Drawing for the job (mm, zero at the part's lowest x, y, z). Coordinates: 2 decimals unless noted, no trailing zeros. Write each loop counter-clockwise with the first axis right and the second up, starting at its lowest first coordinate (ties: lowest second). Pieces come first, ordered by that corner, then holes. Notation, with made-up numbers: M 31,42.25 L 81,42.25 A23 ccw 81,77.25 Z; hole C 67.25,24.5 d6. An arc over 180 degrees is marked long. Put each result on its own line as item: value. Start each with the question number.
Q1. Cut at B-B (x = 81). Write the cut outline in (y, z).
Q2. Cut at A-A (z = 70). Write the cut outline in (x, y).
Q3. Drill centre lines: line 1 along X through (y, z) = (5, 35); line 2 along Z through (x, y) = (208, 3.75); line 3 along Z through (x, y) = (134.57, 4). Where is each one in solid material? Low to high.
Q4. Drop a flat-ended pin along its axis: pin 1 (4 mm diameter, centred on x = 208, z = 35, fed in from +Y). Give the stop position or say it passes through.
Q5. Cut at C-C (x = 134.57). Write the cut outline in (y, z).
Q6. Cut at D-D (z = 35). Write the cut outline in (x, y).
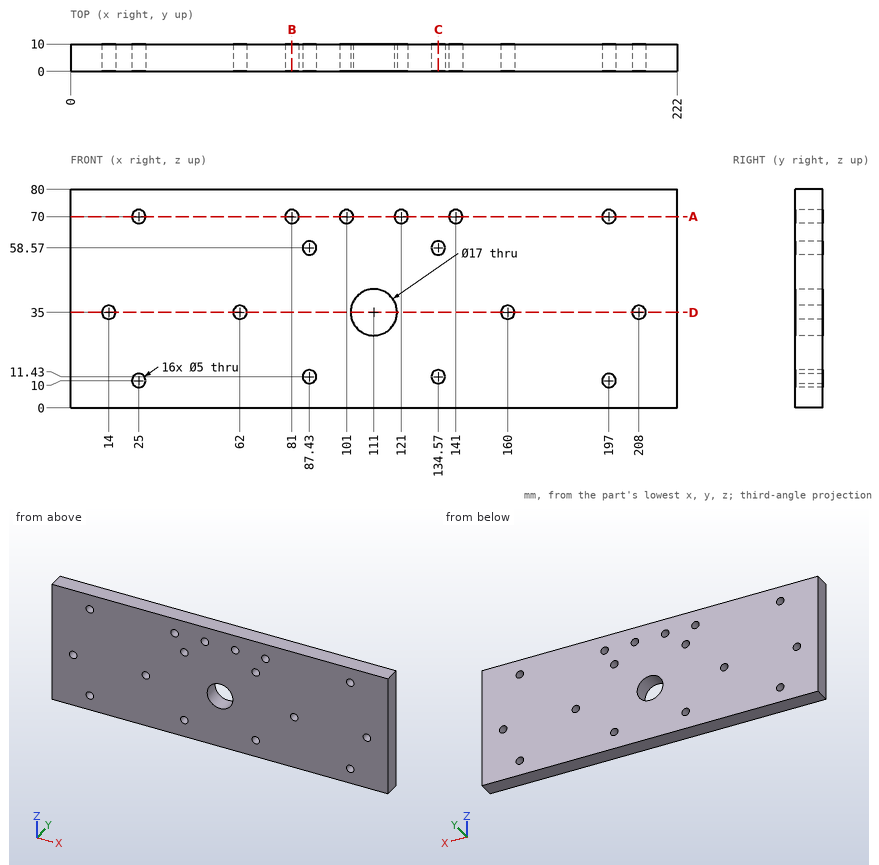
Computed values:
1. outline: M 0,0 L 10,0 L 10,67.5 L 0,67.5 Z; M 0,72.5 L 10,72.5 L 10,80 L 0,80 Z
2. outline: M 0,0 L 22.5,0 L 22.5,10 L 0,10 Z; M 27.5,0 L 78.5,0 L 78.5,10 L 27.5,10 Z; M 83.5,0 L 98.5,0 L 98.5,10 L 83.5,10 Z; M 103.5,0 L 118.5,0 L 118.5,10 L 103.5,10 Z; M 123.5,0 L 138.5,0 L 138.5,10 L 123.5,10 Z; M 143.5,0 L 194.5,0 L 194.5,10 L 143.5,10 Z; M 199.5,0 L 222,0 L 222,10 L 199.5,10 Z
3. line 1: 0 to 11.5, 16.5 to 59.5, 64.5 to 102.5, 119.5 to 157.5, 162.5 to 205.5, 210.5 to 222
3. line 2: 0 to 32.5, 37.5 to 80
3. line 3: 0 to 8.93, 13.93 to 56.07, 61.07 to 80
4. pin 1: through
5. outline: M 0,0 L 10,0 L 10,8.93 L 0,8.93 Z; M 0,13.93 L 10,13.93 L 10,56.07 L 0,56.07 Z; M 0,61.07 L 10,61.07 L 10,80 L 0,80 Z
6. outline: M 0,0 L 11.5,0 L 11.5,10 L 0,10 Z; M 16.5,0 L 59.5,0 L 59.5,10 L 16.5,10 Z; M 64.5,0 L 102.5,0 L 102.5,10 L 64.5,10 Z; M 119.5,0 L 157.5,0 L 157.5,10 L 119.5,10 Z; M 162.5,0 L 205.5,0 L 205.5,10 L 162.5,10 Z; M 210.5,0 L 222,0 L 222,10 L 210.5,10 Z
